Read the model definition and answer for the solid it produces. Units are mm, in the model's axes. A direction names the side the tool comes from. Round coordinates to 2 decimals unless told otherwise and drop trailing zeros. Order: outer loops, then holes, each group sorted by start corner. A loop starts at its lowest first (then second) coordinate and runs counter-clockwise, first axis right, second up.
from build123d import *

# Parameters (mm, degrees)
SKETCH1_R           = 6.35
BOSS_EXTRUDE1_DEPTH = 6.35
CUT_EXTRUDE1_REACH  = 259.643
SKETCH2_W           = 7.108529786
SKETCH2_H           = 8.352611846


with BuildPart() as part:
    # Sketch1 → Boss-Extrude1 (new body)
    with BuildSketch(Plane.XY):
        with BuildLine():
            Line((6.35, 10.998522628), (69.394090512, -25.4))
            Line((69.394090512, -25.4), (169.571649488, -25.4))
            Line((169.571649488, -25.4), (232.61574, 10.998522628))
            ThreePointArc((232.61574, 10.998522628), (249.964262628, 6.35), (245.31574, -10.998522628))
            Line((245.31574, -10.998522628), (169.435593158, -54.807945834))
            Line((169.435593158, -54.807945834), (69.530146842, -54.807945834))
            Line((69.530146842, -54.807945834), (-6.35, -10.998522628))
            ThreePointArc((-6.35, -10.998522628), (-10.998522628, 6.35), (6.35, 10.998522628))
        make_face()
        Circle(SKETCH1_R, mode=Mode.SUBTRACT)
        with Locations((238.96574, 0)):
            Circle(SKETCH1_R, mode=Mode.SUBTRACT)
    extrude(amount=BOSS_EXTRUDE1_DEPTH)

    # Sketch2 → Cut-Extrude1 (cut, up to next)
    with BuildSketch(Plane.XY.offset(6.35), mode=Mode.PRIVATE) as cut_extrude1_sk1:
        with Locations((119.550898165, -40.103972917)):
            Rectangle(SKETCH2_W, SKETCH2_H)
    cut_extrude1_tool1 = extrude(cut_extrude1_sk1.sketch, amount=-CUT_EXTRUDE1_REACH, mode=Mode.PRIVATE) & part.part
    add(cut_extrude1_tool1.solids().sort_by_distance((119.550898, -40.103973, 6.35))[0], mode=Mode.SUBTRACT)


solid = part.part
Q1. Straight lines are drawn through the part: probe 1 along Y at (x, z) = (117.5, 1); probe 2 along X at (y, z) = (-3.5, 4.75); probe 3 along Y at (x, z) = (71.5, 5.5). For each, find the intervals that lie inside material, in ascending order.
Outcome:
probe 1: y = -54.81 to -44.28, -35.93 to -25.4
probe 2: x = -12.21 to -5.3, 5.3 to 31.46, 207.5 to 233.67, 244.26 to 251.17
probe 3: y = -54.81 to -25.4
Q2. A cutting plane is placed at C-C, the plane x = 0. Give the vertices of the cut face in (y, z).
Outcome:
outline: (-14.66, 0) - (-6.35, 0) - (-6.35, 6.35) - (-14.66, 6.35) - close; (6.35, 0) - (12.7, 0) - (12.7, 6.35) - (6.35, 6.35) - close
Q3. A cutting plane is placed at D-D, the plane y = 0. Give the vertices of the cut face in (x, z), plus the area to 3 significant figures.
Outcome:
outline: (-12.7, 0) - (-6.35, 0) - (-6.35, 6.35) - (-12.7, 6.35) - close; (6.35, 0) - (25.4, 0) - (25.4, 6.35) - (6.35, 6.35) - close; (213.57, 0) - (232.62, 0) - (232.62, 6.35) - (213.57, 6.35) - close; (245.32, 0) - (251.67, 0) - (251.67, 6.35) - (245.32, 6.35) - close
area: 323 mm2
Q4. A cutting plane is placed at B-B, the plane y = -22. Give the vertices of the cut face in (x, z).
Outcome:
outline: (12.71, 0) - (63.51, 0) - (63.51, 6.35) - (12.71, 6.35) - close; (175.46, 0) - (226.26, 0) - (226.26, 6.35) - (175.46, 6.35) - close
Q5. For faces 1 (the face through (123.105, -40, 3)), 2 (the face through (207.9, -32.6, 3.1)), 3 (the face through (119, -25.4, 3)), determine the directions among +Z, -Z, +X, -X, +Y, -Y from which every point of the face is accessible in a straight line to the end or side of a thin tool.
Outcome:
face 1: +Z, -Z
face 2: +Z, -Z, +X, -Y
face 3: +Z, -Z, +Y
Q6. Flat-ended cylindrical pins translate along their axes: pin 1 (3 mm diameter, centred on x = 120.5, z = 3.5, fed in from +Y); pin 2 (1.9 mm diameter, centred on y = -38.5, z = 3.5, fed in from -X); pin 3 (3 mm diameter, centred on x = 207, z = 4, fed in from -Y). Find the tip coordinate at first contact, or state that the pin passes through.
Outcome:
pin 1: stops at y = -25.4
pin 2: stops at x = 39.64
pin 3: stops at y = -33.99
Q7. A cutting plane is placed at A-A, the plane z = 1. Give the vertices of the cut face in (x, y), plus the area to 3 significant figures.
Outcome:
outline: (-6.35, -11) - (69.53, -54.81) - (169.44, -54.81) - (245.32, -11) arc R12.7 ccw to (232.62, 11) - (169.57, -25.4) - (69.39, -25.4) - (6.35, 11) arc R12.7 ccw to start; hole circle Ø12.7 at (0, 0); hole (116, -44.28) - (123.11, -44.28) - (123.11, -35.93) - (116, -35.93) - close; hole circle Ø12.7 at (238.97, 0)
area: 7,210 mm2
Q8. For a pull along Y with two mould halves and no side action, classify faces 4 (the face through (249.82, 6.59, 3.13)), 5 (the face through (245.02, 1.91, 3.13)), 6 (the face through (120, -35.928, 3)), 7 (the face through (121, -28, 6.35)) as released by +Y, released by -Y, zero draft, split by the parting line, or undercut.
Outcome:
face 4: split by the parting line
face 5: undercut
face 6: undercut
face 7: zero draft
